The drawing under review shows one solid part. Ordinate dimensions are in mm from its lowest x, y, z. Coordinates: 2 decimals unless noted, no trailing zeros. Order: outer loops, then holes, each group sorted by start corner. A loop starts at its lowest first (then second) coordinate and runs counter-clockwise, first axis right, second up.
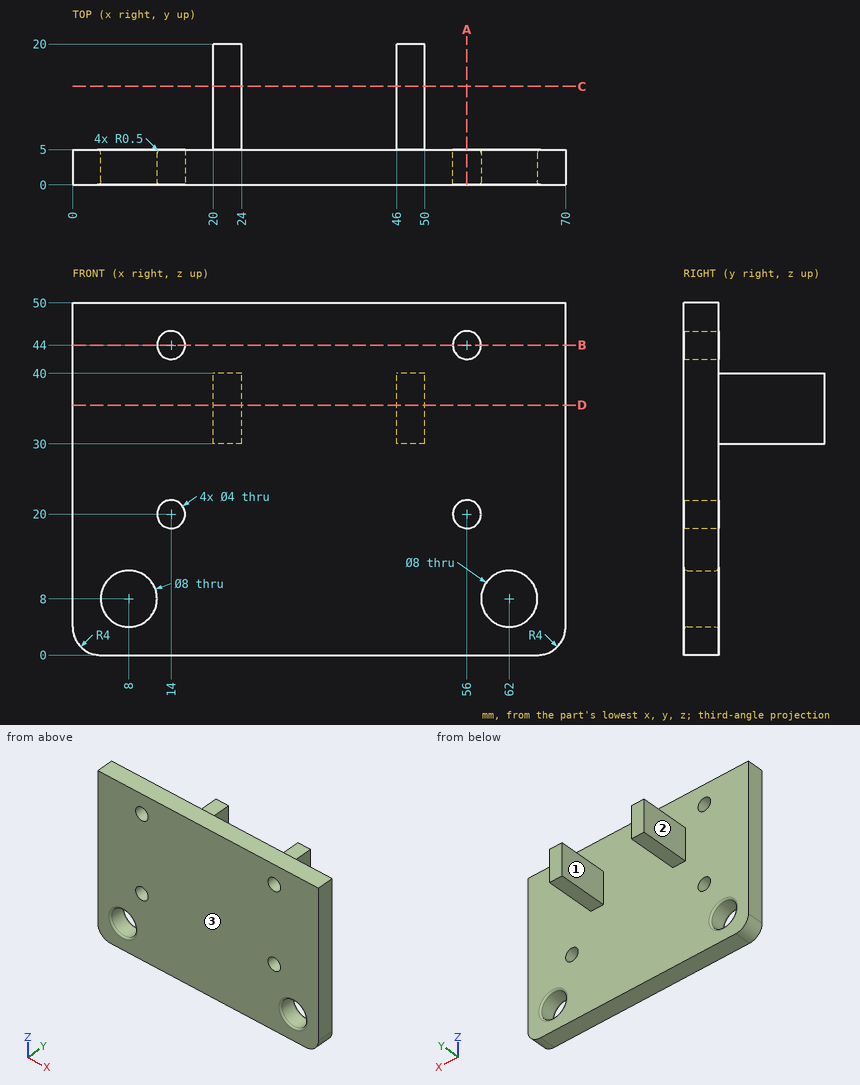
(1) Wall thickness on line 1 (Z direction, x = 14, y = 3.15); line 2 (X direction, y = 16.25, z = 38); line 3 (Z direction, x = 62, y = 3): over which ranges is each line inside the solid? List them lowest first.
(2) Consider section B-B (z = 44). Give the boundary of the cut face in (x, y), then the cut area to 3 significant figures.
(3) Consider section C-C (y = 14). Give the boundary of the cut face in (x, z).
(4) Consider section D-D (z = 35.5). Give the boundary of the cut face in (x, y).
(5) The part is to be moulded in two halves that separate along X. For the marked faces 1, 2 and 3, say which applies: +X half, -X half, draft (parallel to the pull), parting line (faces both ways), or undercut.
(6) Consider section A-A (x = 56). Give the boundary of the cut face in (y, z), then the cut area to 3 significant figures.
(7) Insertion check: pin 1 Ø6 at (x, z) = (57.5, 38) entering from +Y; pin 2 Ø2 at (x, y) = (21, 12.5) entering from +Z; pin 3 Ø4 at (y, z) = (17, 32.5) entering from +X; pin 4 Ø10 at (x, y) = (12.5, 11) entering from -Z. Each pin has a flat end and moves straight along its axis. Give the tip position at first contact, or say it passes through.
Findings:
1. line 1: z = 0 to 18, 22 to 42, 46 to 50
1. line 2: x = 20 to 24, 46 to 50
1. line 3: z = 0 to 4, 12 to 50
2. outline: (0, 0) - (12, 0) - (12, 5) - (0, 5) - close; (16, 0) - (54, 0) - (54, 5) - (16, 5) - close; (58, 0) - (70, 0) - (70, 5) - (58, 5) - close
2. area: 310 mm2
3. outline: (20, 30) - (24, 30) - (24, 40) - (20, 40) - close; (46, 30) - (50, 30) - (50, 40) - (46, 40) - close
4. outline: (0, 0) - (70, 0) - (70, 5) - (50, 5) - (50, 20) - (46, 20) - (46, 5) - (24, 5) - (24, 20) - (20, 20) - (20, 5) - (0, 5) - close
5. face 1: undercut
5. face 2: -X half
5. face 3: draft
6. outline: (0, 0) - (5, 0) - (5, 18) - (0, 18) - close; (0, 22) - (5, 22) - (5, 42) - (0, 42) - close; (0, 46) - (5, 46) - (5, 50) - (0, 50) - close
6. area: 210 mm2
7. pin 1: stops at y = 5
7. pin 2: stops at z = 40
7. pin 3: stops at x = 50
7. pin 4: passes through
